Can you work these out from the model? Positions are in its coordinate system, mm. Coordinates: 2 decimals unless noted, no trailing zeros. Order: outer loops, then holes, each group sorted by start corner. A loop starts at its lowest first (then second) coordinate and runs counter-clockwise, first axis right, second up. Notation, with made-up numbers: (4.25, 18) -> (50.25, 18) arc R22 cw to (50.25, 39) -> close; hole circle Ø6 at (-9.75, 32). An arc over 180 degrees is marked (long way). Return JSON: item names as keys, results as strings. Group by question number.
1) If we section it at A-A, the plane y = -10: Please give me the cut outline in (x, z), then the cut area to 3 significant figures.
2) For pin 1 (9 mm diameter, centred on x = 10, y = -10, fed in from +Z); pin 2 (5.5 mm diameter, centred on x = 288, y = -49.5, fed in from -Z); pin 3 (4.5 mm diameter, centred on x = 270, z = 0, fed in from -Y); pin 4 (2.5 mm diameter, centred on x = 45, y = -20, fed in from -Z), each with a flat end and sliding along its axis, tell me the tip position at first contact or that it passes through.
3) If we section it at B-B, the plane x = 290: Please give me the cut outline in (y, z).
4) If I drill on probe 1 along X at (y, z) = (-20.5, -1.75); probe 2 along X at (y, z) = (-49.5, 0); probe 3 along Y at (x, z) = (10, 3.95), over which ranges is the centre line in solid material (lowest first)? Write a range as from..to.
from build123d import *

# Parameters (mm, degrees)
SKETCH_1_W                = 300
SKETCH_1_H                = 60
EXTRUDE_1_DEPTH           = 5
HOLE_WIZARD_M6_1_D        = 5
HOLE_WIZARD_M6_1_DEPTH    = 15
HOLE_WIZARD_M6_1_TIP      = 1.502151548
HOLE_WIZARD_1_D           = 6.6
HOLE_WIZARD_1_CBORE_D     = 11
HOLE_WIZARD_1_CBORE_DEPTH = 6.8
HOLE_WIZARD_M5_1_D        = 4.2


with BuildPart() as part:
    # 草图1 → 凸台-拉伸1 (new body, symmetric)
    with BuildSketch(Plane.XY):
        with Locations((150, -30)):
            Rectangle(SKETCH_1_W, SKETCH_1_H)
    extrude(amount=EXTRUDE_1_DEPTH, both=True)

    # M6 螺纹孔1
    with Locations(Plane(origin=(30, -60, 0), x_dir=(0, 0, -1), z_dir=(0, -1, 0))):
        with Locations((0, 0), (0, 240), (0, 120)):
            Hole(HOLE_WIZARD_M6_1_D / 2, depth=HOLE_WIZARD_M6_1_DEPTH)
            with Locations((0, 0, -(HOLE_WIZARD_M6_1_DEPTH + HOLE_WIZARD_M6_1_TIP / 2))):  # 118° drill point
                Cone(0, HOLE_WIZARD_M6_1_D / 2, HOLE_WIZARD_M6_1_TIP, mode=Mode.SUBTRACT)

    # 打孔尺寸(%根据)内六角圆柱头螺钉的类型1 (through all)
    with Locations(Plane(origin=(10, -10, -5), x_dir=(-1, 0, 0), z_dir=(0, 0, -1))):
        with Locations((0, 0), (0, -40), (-280, 0), (-280, -40)):
            CounterBoreHole(HOLE_WIZARD_1_D / 2, HOLE_WIZARD_1_CBORE_D / 2, HOLE_WIZARD_1_CBORE_DEPTH)

    # M5 螺纹孔1 (through all)
    with Locations(Plane(origin=(45, -20, -5), x_dir=(-1, 0, 0), z_dir=(0, 0, -1))):
        with Locations((0, 0), (0, -20)):
            hole_wizard_m5_1 = Hole(HOLE_WIZARD_M5_1_D / 2)

    # 镜向1: M5 螺纹孔1 across plane
    add(hole_wizard_m5_1.mirror(Plane(origin=(150, 0, 0), x_dir=(0, 0, 1), z_dir=(1, 0, 0))), mode=Mode.SUBTRACT)


solid = part.part
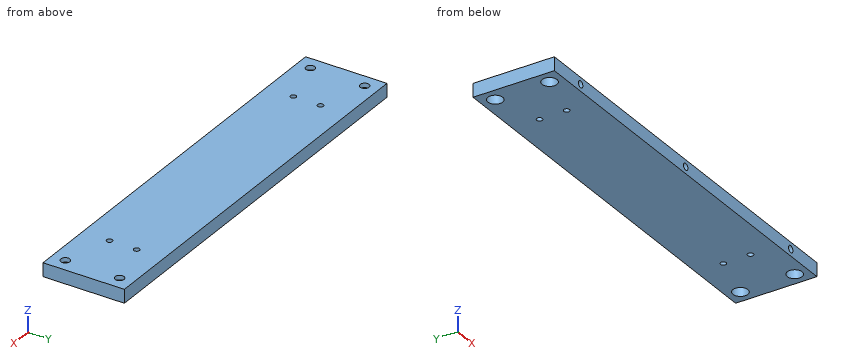
Result sheet:
{
 "1": {"outline": "(0, -5) -> (4.5, -5) -> (4.5, 1.8) -> (6.7, 1.8) -> (6.7, 5) -> (0, 5) -> close; (13.3, 1.8) -> (15.5, 1.8) -> (15.5, -5) -> (284.5, -5) -> (284.5, 1.8) -> (286.7, 1.8) -> (286.7, 5) -> (13.3, 5) -> close; (293.3, 1.8) -> (295.5, 1.8) -> (295.5, -5) -> (300, -5) -> (300, 5) -> (293.3, 5) -> close", "area": "2,810 mm2"},
 "2": {"pin 1": "stops at z = 5", "pin 2": "stops at z = 1.8", "pin 3": "stops at y = -44.85", "pin 4": "passes through"},
 "3": {"outline": "(-60, -5) -> (-55.5, -5) -> (-55.5, 1.8) -> (-53.3, 1.8) -> (-53.3, 5) -> (-60, 5) -> close; (-46.7, 1.8) -> (-44.5, 1.8) -> (-44.5, -5) -> (-15.5, -5) -> (-15.5, 1.8) -> (-13.3, 1.8) -> (-13.3, 5) -> (-46.7, 5) -> close; (-6.7, 1.8) -> (-4.5, 1.8) -> (-4.5, -5) -> (0, -5) -> (0, 5) -> (-6.7, 5) -> close"},
 "4": {"probe 1": "x = 0..42.96, 47.04..252.96, 257.04..300", "probe 2": "x = 0..4.52, 15.48..27.5, 32.5..147.5, 152.5..267.5, 272.5..284.52, 295.48..300", "probe 3": "y = -60..-53.3, -46.7..-13.3, -6.7..0"}
}
